from build123d import *

# Parameters (mm, degrees)
ESQUISSE1_R                  = 4.5
BOSS_EXTRU_1_DEPTH           = 3
BOSS_EXTRU_2_START           = -0.5
ESQUISSE2_R                  = 0.75
BOSS_EXTRU_2_DEPTH           = 2
R_P_TITION_CIRCULAIRE1_COUNT = 2
ESQUISSE5_R                  = 4.5
ESQUISSE5_R_2                = 1.4
BOSS_EXTRU_4_DEPTH           = 0.7
ESQUISSE6_R                  = 4.5
ESQUISSE6_R_2                = 3
BOSS_EXTRU_5_DEPTH           = 0.8
ESQUISSE7_R                  = 3.75
ESQUISSE7_R_2                = 3
BOSS_EXTRU_6_DEPTH           = 0.8


with BuildPart() as part:
    # Esquisse1 → Boss.-Extru.1 (new body)
    with BuildSketch(Plane.XY):
        Circle(ESQUISSE1_R)
        Polygon((2.011577371, -1.550856692), (2.011577371, -2.011577371), (1.550856692, -2.011577371), (1.541643286, -2.018647066), (1.4224, -2.463669069), (0.977377998, -2.344425783), (0.966648759, -2.348869979), (0.73628842, -2.747865791), (0.337292608, -2.517505451), (0.325778716, -2.519021284), (0, -2.8448), (-0.325778716, -2.519021284), (-0.337292608, -2.517505451), (-0.73628842, -2.747865791), (-0.966648759, -2.348869979), (-0.977377998, -2.344425783), (-1.4224, -2.463669069), (-1.541643286, -2.018647066), (-1.550856692, -2.011577371), (-2.011577371, -2.011577371), (-2.011577371, -1.550856692), (-2.018647066, -1.541643286), (-2.463669069, -1.4224), (-2.344425783, -0.977377998), (-2.348869979, -0.966648759), (-2.747865791, -0.73628842), (-2.517505451, -0.337292608), (-2.519021284, -0.325778716), (-2.8448, 0), (-2.519021284, 0.325778716), (-2.517505451, 0.337292608), (-2.747865791, 0.73628842), (-2.348869979, 0.966648759), (-2.344425783, 0.977377998), (-2.463669069, 1.4224), (-2.018647066, 1.541643286), (-2.011577371, 1.550856692), (-2.011577371, 2.011577371), (-1.550856692, 2.011577371), (-1.541643286, 2.018647066), (-1.4224, 2.463669069), (-0.977377998, 2.344425783), (-0.966648759, 2.348869979), (-0.73628842, 2.747865791), (-0.337292608, 2.517505451), (-0.325778716, 2.519021284), (0, 2.8448), (0.325778716, 2.519021284), (0.337292608, 2.517505451), (0.73628842, 2.747865791), (0.966648759, 2.348869979), (0.977377998, 2.344425783), (1.4224, 2.463669069), (1.541643286, 2.018647066), (1.550856692, 2.011577371), (2.011577371, 2.011577371), (2.011577371, 1.550856692), (2.018647066, 1.541643286), (2.463669069, 1.4224), (2.344425783, 0.977377998), (2.348869979, 0.966648759), (2.747865791, 0.73628842), (2.517505451, 0.337292608), (2.519021284, 0.325778716), (2.8448, 0), (2.519021284, -0.325778716), (2.517505451, -0.337292608), (2.747865791, -0.73628842), (2.348869979, -0.966648759), (2.344425783, -0.977377998), (2.463669069, -1.4224), (2.018647066, -1.541643286), align=None, mode=Mode.SUBTRACT)
    extrude(amount=BOSS_EXTRU_1_DEPTH)

    # Esquisse2 → Boss.-Extru.2 (add)
    with BuildSketch(Plane.XY.offset(3).offset(BOSS_EXTRU_2_START)):
        with BuildLine():
            Line((-14.844827586, 2.476104589), (-0.620689655, 4.45698826))
            ThreePointArc((-0.620689655, 4.45698826), (-4.5, 0), (-0.620689655, -4.45698826))
            Line((-0.620689655, -4.45698826), (-14.844827586, -2.476104589))
            ThreePointArc((-14.844827586, -2.476104589), (-17, 0), (-14.844827586, 2.476104589))
        make_face()
        with Locations((-14.5, 0)):
            Circle(ESQUISSE2_R, mode=Mode.SUBTRACT)
        with Locations((-12, 0)):
            Circle(ESQUISSE2_R, mode=Mode.SUBTRACT)
        with Locations((-9.5, 0)):
            Circle(ESQUISSE2_R, mode=Mode.SUBTRACT)
    boss_extru_2 = extrude(amount=BOSS_EXTRU_2_DEPTH)

    # Répétition circulaire1: Boss.-Extru.2 ×2 about axis
    r_p_tition_circulaire1_axis = Axis((0, 0, 0), (0, 0, 1))
    for i in range(1, R_P_TITION_CIRCULAIRE1_COUNT):
        add(boss_extru_2.rotate(r_p_tition_circulaire1_axis, i * 360 / R_P_TITION_CIRCULAIRE1_COUNT))

    # Esquisse5 → Boss.-Extru.4 (add)
    with BuildSketch(Plane.XY.offset(3)):
        Circle(ESQUISSE5_R)
        Circle(ESQUISSE5_R_2, mode=Mode.SUBTRACT)
    extrude(amount=BOSS_EXTRU_4_DEPTH)

    # Esquisse6 → Boss.-Extru.5 (add)
    with BuildSketch(Plane.XY.offset(3.7)):
        Circle(ESQUISSE6_R)
        Circle(ESQUISSE6_R_2, mode=Mode.SUBTRACT)
    extrude(amount=BOSS_EXTRU_5_DEPTH)

    # Esquisse7 → Boss.-Extru.6 (add)
    with BuildSketch(Plane.XY.offset(4.5)):
        Circle(ESQUISSE7_R)
        Circle(ESQUISSE7_R_2, mode=Mode.SUBTRACT)
    extrude(amount=BOSS_EXTRU_6_DEPTH)


solid = part.part
Work out the finished part from the listing and answer in its coordinate system (mm). A direction names the side the tool comes from. Give positions to 0.01 mm unless a question says otherwise; leave off trailing zeros. Order: outer loops, then holes, each group sorted by start corner. A loop starts at its lowest first (then second) coordinate and runs counter-clockwise, first axis right, second up. Notation, with made-up numbers: (37.5, 79.25) - (54.5, 79.25) arc R14 ccw to (54.5, 93.25) - close; hole circle Ø4 at (-32, 75.5). An arc over 180 degrees is marked (long way). Answer as CSV lines item,"result". Start each with the question number.
Q1. The mould has two halves that part along X. Classify faces 1 (the face through (-3, 0, 4)), 2 (the face through (-17, 0, 3)), 3 (the face through (0, -3, 0)): +X half, -X half, draft (parallel to the pull), parting line (faces both ways), or undercut.
Q2. The part is cut by section B-B (x = -12). Write down the section's boundary in (y, z), then the cut area to 3 significant figures.
Q3. The part is cut by section C-C (x = 9.5). Write down the section's boundary in (y, z).
Q4. For faces 4 (the face through (-3.746, 0.165, 4.894)), 5 (the face through (-1.3, 1.3, 3)), 6 (the face through (7.832, -3.453, 3.486)), determine the directions among +Z, -Z, +X, -X, +Y, -Y from which every point of the face is accessible in a straight line to the end or side of a thin tool.
Q5. Find the intervals of material crossed by L1, parallel to Z at x = 1.5, y = -1.5; L2, parallel to Z at x = 7.5, y = 2.75; L3, parallel to X at y = 1, z = 1.3, in increasing order. Write a range as [from, to].
Q6. Given pin 1 Ø1.4 at (x, y) = (-12, 0) entering from +Z; pin 2 Ø5 at (x, y) = (-5, 2) entering from +Z; pin 3 Ø0.5 at (y, z) = (-2, 1) entering from -X; pin 4 Ø4.5 at (x, y) = (-9, 1) entering from -Z, each flat-ended and moving along its own axis, determine where each tip first touches the part or whether it passes through.
Q7. The part is cut by section A-A (z = 4.15). Write down the section's boundary in (x, y).
Check result:
1,face 1,"undercut"
1,face 2,"-X half"
1,face 3,"draft"
2,outline,"(-2.87, 2.5) - (-0.75, 2.5) - (-0.75, 4.5) - (-2.87, 4.5) - close; (0.75, 2.5) - (2.87, 2.5) - (2.87, 4.5) - (0.75, 4.5) - close"
2,area,"8.49 mm²"
3,outline,"(-3.22, 2.5) - (-0.75, 2.5) - (-0.75, 4.5) - (-3.22, 4.5) - close; (0.75, 2.5) - (3.22, 2.5) - (3.22, 4.5) - (0.75, 4.5) - close"
4,face 4,"+Z"
4,face 5,"-Z"
4,face 6,"+Z, -Z, +X, -Y"
5,L1,"z = [3, 3.7]"
5,L2,"z = [2.5, 4.5]"
5,L3,"x = [-4.39, -2.35], [2.35, 4.39]"
6,pin 1,"passes through"
6,pin 2,"stops at z = 5.3"
6,pin 3,"stops at x = -4.15"
6,pin 4,"stops at z = 2.5"
7,outline,"(-14.84, -2.48) - (-0.62, -4.46) arc R4.5 ccw to (0.62, -4.46) - (14.84, -2.48) arc R2.5 ccw to (14.84, 2.48) - (0.62, 4.46) arc R4.5 ccw to (-0.62, 4.46) - (-14.84, 2.48) arc R2.5 ccw to start; hole circle Ø1.5 at (-14.5, 0); hole circle Ø1.5 at (-12, 0); hole circle Ø1.5 at (-9.5, 0); hole circle Ø6 at (0, 0); hole circle Ø1.5 at (9.5, 0); hole circle Ø1.5 at (12, 0); hole circle Ø1.5 at (14.5, 0)"
